Source: CAD feature listing. Evaluate the final solid. Frame: model axes, mm. A direction names the side the tool comes from. Give positions to 0.01 mm unless a question says otherwise; leave off trailing zeros. Loops run counter-clockwise (first coordinate to the right, second up) from the corner with the lowest first, then second, coordinate; pieces in that order, holes last. Notation, with made-up numbers: (64, -6.5) -> (100, -6.5) arc R16 cw to (100, 23.5) -> close; hole circle Ø11 at (-0.5, 19). An arc over 180 degrees is marked (long way). Return JSON: item names as keys, results as strings. Group by question number.
Autodesk Inventor part; units mm, degrees
ref_plane "YZ Plane" through (0, 0, 0) normal (1, 0, 0) x (0, 1, 0)
ref_plane "XZ Plane" through (0, 0, 0) normal (0, 1, 0) x (-1, 0, 0)
ref_plane "XY Plane" through (0, 0, 0) normal (0, 0, 1) x (1, 0, 0)
sketch "Sketch1" plane through (0, 0, 0) normal (0, 0, 1) x (1, 0, 0)
  line L0 (47.0185, 51.5544) -> (-48.0003, 51.5544)
  line L1 (-48.0003, 51.5544) -> (-48.0003, -51.5544)
  line L2 (-48.0003, -51.5544) -> (47.0185, -51.5544)
  line L3 (47.0185, -51.5544) -> (47.0185, 51.5544)
  line L4 (41.2041, -35.74) -> (41.2041, 35.74)
  arc A0 (41.2041, 35.74) -> (31.2041, 45.74) centre (31.2041, 35.74) ccw
  line L5 (31.2041, 45.74) -> (-32.1859, 45.74)
  arc A1 (-32.1859, 45.74) -> (-42.1859, 35.74) centre (-32.1859, 35.74) ccw
  line L6 (-42.1859, 35.74) -> (-42.1859, -35.74)
  arc A2 (-42.1859, -35.74) -> (-32.1859, -45.74) centre (-32.1859, -35.74) ccw
  line L7 (-32.1859, -45.74) -> (31.2041, -45.74)
  arc A3 (31.2041, -45.74) -> (41.2041, -35.74) centre (31.2041, -35.74) ccw
  circle A4 centre (24.0591, 16.9245) radius 1.25
  circle A5 centre (24.0591, -43.0755) radius 1.25
  circle A6 centre (-25.0409, -43.0755) radius 1.25
  circle A7 centre (-25.0409, 16.9245) radius 1.25
  line L8 (25.5091, 38.0745) -> (-26.4909, 38.0745)
  arc A8 (-26.4909, 38.0745) -> (-28.4909, 36.0745) centre (-26.4909, 36.0745) ccw
  line L9 (-28.4909, 36.0745) -> (-28.4909, -44.9255)
  arc A9 (-28.4909, -44.9255) -> (-26.4909, -46.9255) centre (-26.4909, -44.9255) ccw
  line L10 (-26.4909, -46.9255) -> (25.5091, -46.9255)
  arc A10 (25.5091, -46.9255) -> (27.5091, -44.9255) centre (25.5091, -44.9255) ccw
  line L11 (27.5091, -44.9255) -> (27.5091, 36.0745)
  arc A11 (27.5091, 36.0745) -> (25.5091, 38.0745) centre (25.5091, 36.0745) ccw
  point P0 (0, 0)
  dimension "d2" = 5.8144
  dimension "d3" = 5.8144
  dimension "d4" = 5.8144
  dimension "d5" = 5.8144
extrude "Extrusion1" add sketch "Sketch1" along normal blind 3 contours L3 L2 L1 L0 | A3 L7 A10 L11 A11 L8 A8 L9 A9 A2 L6 A1 L5 A0 L4 | A10 L10 A9 L7 | L7 A9 L9 A8 L8 A11 L11 A10 | A4 | A5 | A6 | A7
sketch "Sketch3" plane through (0, 0, 0) normal (0, 0, -1) x (-1, 0, 0)
  line L0 (-41.2041, 35.74) -> (-41.2041, -35.74)
  arc A0 (-41.2041, -35.74) -> (-31.2041, -45.74) centre (-31.2041, -35.74) ccw
  line L1 (-31.2041, -45.74) -> (32.1859, -45.74)
  arc A1 (32.1859, -45.74) -> (42.1859, -35.74) centre (32.1859, -35.74) ccw
  line L2 (42.1859, -35.74) -> (42.1859, 35.74)
  arc A2 (42.1859, 35.74) -> (32.1859, 45.74) centre (32.1859, 35.74) ccw
  line L3 (32.1859, 45.74) -> (-31.2041, 45.74)
  arc A3 (-31.2041, 45.74) -> (-41.2041, 35.74) centre (-31.2041, 35.74) ccw
  line L4 (43.1859, 43.5544) -> (46.1859, 43.5544)
  line L5 (46.1859, 43.5544) -> (46.1859, -43.5544)
  line L6 (46.1859, -43.5544) -> (43.1859, -43.5544)
  line L7 (43.1859, -43.5544) -> (43.1859, 43.5544)
  line L8 (-42.2041, 43.5544) -> (-45.2041, 43.5544)
  line L9 (-45.2041, 43.5544) -> (-45.2041, -43.5544)
  line L10 (-45.2041, -43.5544) -> (-42.2041, -43.5544)
  line L11 (-42.2041, -43.5544) -> (-42.2041, 43.5544)
  line L12 (40.0003, 49.74) -> (-39.0185, 49.74)
  line L13 (-39.0185, 49.74) -> (-39.0185, 46.74)
  line L14 (-39.0185, 46.74) -> (40.0003, 46.74)
  line L15 (40.0003, 46.74) -> (40.0003, 49.74)
  line L16 (40.0003, -46.74) -> (-39.0185, -46.74)
  line L17 (-39.0185, -46.74) -> (-39.0185, -49.74)
  line L18 (-39.0185, -49.74) -> (40.0003, -49.74)
  line L19 (40.0003, -49.74) -> (40.0003, -46.74)
  line L20 (-47.0185, 51.5544) -> (48.0003, 51.5544)
  line L21 (48.0003, 51.5544) -> (48.0003, -51.5544)
  line L22 (48.0003, -51.5544) -> (-47.0185, -51.5544)
  line L23 (-47.0185, -51.5544) -> (-47.0185, 51.5544)
  point P0 (0, 0)
  dimension "d20" = 3
  dimension "d21" = 1
  dimension "d24" = 3
  dimension "d25" = 1
  dimension "d28" = 3
  dimension "d29" = 1
  dimension "d34" = 1
  dimension "d35" = 3
  dimension "d78" = 8
  dimension "d79" = 8
  dimension "d80" = 8
  dimension "d81" = 8
  dimension "d82" = 8
  dimension "d83" = 8
  dimension "d84" = 8
  dimension "d85" = 8
extrude "Extrusion2" add sketch "Sketch3" along normal blind 5 contours L4 L5 L6 L7 | L11 L10 L9 L8 | L15 L14 L13 L12 | L19 L18 L17 L16
sketch "Sketch6" plane through (0, 0, 0) normal (0, 0, -1) x (-1, 0, 0)
  line L0 (48.0003, 51.5544) -> (48.0003, -51.5544)
  line L1 (48.0003, 51.5544) -> (40.0003, 51.5544)
  line L2 (40.0003, 51.5544) -> (40.0003, 43.5544)
  line L3 (40.0003, 43.5544) -> (48.0003, 43.5544)
  line L4 (48.0003, 43.5544) -> (48.0003, 51.5544)
  line L5 (48.0003, -51.5544) -> (40.0003, -51.5544)
  line L6 (40.0003, -51.5544) -> (40.0003, -43.5544)
  line L7 (40.0003, -43.5544) -> (48.0003, -43.5544)
  line L8 (48.0003, -43.5544) -> (48.0003, -51.5544)
  line L9 (48.0003, -51.5544) -> (-47.0185, -51.5544)
  line L10 (-47.0185, -51.5544) -> (-39.0185, -51.5544)
  line L11 (-39.0185, -51.5544) -> (-39.0185, -43.5544)
  line L12 (-39.0185, -43.5544) -> (-47.0185, -43.5544)
  line L13 (-47.0185, -43.5544) -> (-47.0185, -51.5544)
  line L14 (-47.0185, 51.5544) -> (48.0003, 51.5544)
  line L15 (-47.0185, 51.5544) -> (-39.0185, 51.5544)
  line L16 (-39.0185, 51.5544) -> (-39.0185, 43.5544)
  line L17 (-39.0185, 43.5544) -> (-47.0185, 43.5544)
  line L18 (-47.0185, 43.5544) -> (-47.0185, 51.5544)
  point P0 (0, 0)
  dimension "d38" = 8
  dimension "d39" = 8
  dimension "d40" = 8
  dimension "d41" = 8
  dimension "d42" = 8
  dimension "d43" = 8
  dimension "d44" = 8
  dimension "d45" = 8
extrude "Extrusion3" add sketch "Sketch6" along normal blind 6
sketch "Sketch7" plane through (0, 0, 3) normal (0, 0, 1) x (1, 0, 0)
  line L0 (47.0185, -51.5544) -> (47.0185, 51.5544)
  line L1 (47.0185, 51.5544) -> (40.0185, 51.5544)
  line L2 (40.0185, 51.5544) -> (40.0185, 44.5544)
  line L3 (40.0185, 44.5544) -> (47.0185, 44.5544)
  line L4 (47.0185, 44.5544) -> (47.0185, 51.5544)
  line L5 (47.0185, -51.5544) -> (40.0185, -51.5544)
  line L6 (40.0185, -51.5544) -> (40.0185, -44.5544)
  line L7 (40.0185, -44.5544) -> (47.0185, -44.5544)
  line L8 (47.0185, -44.5544) -> (47.0185, -51.5544)
  line L9 (-48.0003, 51.5544) -> (-48.0003, -51.5544)
  line L10 (-48.0003, -51.5544) -> (-41.0003, -51.5544)
  line L11 (-41.0003, -51.5544) -> (-41.0003, -44.5544)
  line L12 (-41.0003, -44.5544) -> (-48.0003, -44.5544)
  line L13 (-48.0003, -44.5544) -> (-48.0003, -51.5544)
  line L14 (-48.0003, 51.5544) -> (-41.0003, 51.5544)
  line L15 (-41.0003, 51.5544) -> (-41.0003, 44.5544)
  line L16 (-41.0003, 44.5544) -> (-48.0003, 44.5544)
  line L17 (-48.0003, 44.5544) -> (-48.0003, 51.5544)
  point P0 (0, 0)
  dimension "d48" = 7
  dimension "d49" = 7
  dimension "d50" = 7
  dimension "d51" = 7
  dimension "d52" = 7
  dimension "d53" = 7
  dimension "d54" = 7
  dimension "d55" = 7
extrude "Extrusion4" cut sketch "Sketch7" against normal blind 6
sketch "Sketch8" plane through (0, 0, -3) normal (0, 0, 1) x (1, 0, 0)
  circle A0 centre (43.5185, 48.0544) radius 1.5
  circle A1 centre (43.5185, -48.0544) radius 1.5
  circle A2 centre (-44.5003, -48.0544) radius 1.5
  circle A3 centre (-44.5003, 48.0544) radius 1.5
  line L0 (47.0185, 51.5544) -> (47.0185, 44.5544)
  line L1 (40.0185, 51.5544) -> (47.0185, 51.5544)
  line L2 (47.0185, -44.5544) -> (47.0185, -51.5544)
  line L3 (47.0185, -51.5544) -> (40.0185, -51.5544)
  line L4 (-48.0003, -51.5544) -> (-48.0003, -44.5544)
  line L5 (-41.0003, -51.5544) -> (-48.0003, -51.5544)
  line L6 (-48.0003, 44.5544) -> (-48.0003, 51.5544)
  line L7 (-48.0003, 51.5544) -> (-41.0003, 51.5544)
  point P0 (0, 0)
  dimension "d58" = 3
  dimension "d59" = 3
  dimension "d60" = 3
  dimension "d61" = 3
  dimension "d62" = 3.5
  dimension "d63" = 3.5
  dimension "d64" = 3.5
  dimension "d65" = 3.5
  dimension "d66" = 3.5
  dimension "d67" = 3.5
  dimension "d68" = 3.5
  dimension "d69" = 3.5
extrude "Extrusion5" cut sketch "Sketch8" against normal up to next
sketch "Sketch9" plane through (0, 0, 3) normal (0, 0, 1) x (1, 0, 0)
  circle A0 centre (24.0497, -29.5956) radius 1.25
  circle A1 centre (-25.0503, -29.5956) radius 1.25
  line L0 (25.4997, 51.5544) -> (-26.5003, 51.5544)
  arc A2 (-26.5003, 51.5544) -> (-28.5003, 49.5544) centre (-26.5003, 49.5544) ccw
  line L1 (-28.5003, 49.5544) -> (-28.5003, -31.4456)
  arc A3 (-28.5003, -31.4456) -> (-26.5003, -33.4456) centre (-26.5003, -31.4456) ccw
  line L2 (-26.5003, -33.4456) -> (25.4997, -33.4456)
  arc A4 (25.4997, -33.4456) -> (27.4997, -31.4456) centre (25.4997, -31.4456) ccw
  line L3 (27.4997, -31.4456) -> (27.4997, 49.5544)
  arc A5 (27.4997, 49.5544) -> (25.4997, 51.5544) centre (25.4997, 49.5544) ccw
  circle A6 centre (24.0497, -29.5956) radius 1.5
  circle A7 centre (-25.0503, -29.5956) radius 1.5
  circle A8 centre (24.0497, 27.9044) radius 1.25
  circle A9 centre (24.0497, -29.5956) radius 1.25
  circle A10 centre (-25.0503, -29.5956) radius 1.25
  circle A11 centre (-25.0503, 27.9044) radius 1.25
  line L4 (25.4997, 51.5544) -> (-26.5003, 51.5544)
  arc A12 (-26.5003, 51.5544) -> (-28.5003, 49.5544) centre (-26.5003, 49.5544) ccw
  line L5 (-28.5003, 49.5544) -> (-28.5003, -31.4456)
  arc A13 (-28.5003, -31.4456) -> (-26.5003, -33.4456) centre (-26.5003, -31.4456) ccw
  line L6 (-26.5003, -33.4456) -> (25.4997, -33.4456)
  arc A14 (25.4997, -33.4456) -> (27.4997, -31.4456) centre (25.4997, -31.4456) ccw
  line L7 (27.4997, -31.4456) -> (27.4997, 49.5544)
  arc A15 (27.4997, 49.5544) -> (25.4997, 51.5544) centre (25.4997, 49.5544) ccw
  circle A16 centre (24.0497, 27.9044) radius 1.5
  circle A17 centre (-25.0503, 27.9044) radius 1.5
  point P0 (0, 0)
  dimension "d73" = 3
  dimension "d74" = 3
  dimension "d86" = 3
  dimension "d87" = 3
extrude "Extrusion6" cut sketch "Sketch9" against normal up to next contours A0 | A1 | A6 | A7 | A8 | A11 | A16 | A17
equation "\"d3\" = d2"
equation "\"d4\" = d2"
equation "\"d5\" = d2"
equation "\"d39\" = d38"
equation "\"d40\" = d38"
equation "\"d41\" = d38"
equation "\"d42\" = d38"
equation "\"d43\" = d38"
equation "\"d44\" = d38"
equation "\"d45\" = d38"
equation "\"d49\" = d48"
equation "\"d50\" = d48"
equation "\"d51\" = d48"
equation "\"d52\" = d48"
equation "\"d53\" = d48"
equation "\"d54\" = d48"
equation "\"d55\" = d48"
equation "\"d62\" = 0.5 * d48"
equation "\"d63\" = d62"
equation "\"d64\" = d62"
equation "\"d65\" = d62"
equation "\"d66\" = d62"
equation "\"d67\" = d62"
equation "\"d68\" = d62"
equation "\"d69\" = d62"
equation "\"d74\" = d73"
equation "\"d86\" = d73"
equation "\"d87\" = d73"
properties part number "akksi-raspi"
1) Contact query for flat-ended pins moving along their axis: P1, Ø1.8, axis at x = 43.52, y = -48.05, coming from the +Z side; P2, Ø1, axis at y = -28, z = -2, coming from the -X side; P3, Ø3.5, axis at x = -17, y = -48.5, coming from the -Z side; P4, Ø2, axis at x = -35, z = -4, coming from the -Y side. Output: stop coordinate, or through.
2) Material intervals for line 1 (X direction, y = 5, z = -1); line 2 (Y direction, x = 18, z = -4.75); line 3 (Y direction, x = 23, z = 2), sorted ascending.
3) Reachability of faces 4 (the face through (43, 50, -3)), 5 (the face through (42.204, -1, -2)), 6 (the face through (0, -49.74, -2)) from +Z, -Z, +X, -X, +Y, -Y: full face, straight path, thin tool, end or side. Return the list, or none.
4) Cut plane B-B on x = 6.5. Return loops of the section in (y, z), then the cut area to 3 significant figures.
5) Cut plane A-A on y = -20.5. Return loops of the section in (x, z).
6) Cut plane C-C on z = 1.5. Return loops of the section in (x, y), then the cut area to 3 significant figures.
7) Mould query, pull axis Y, two halves, no side actions, for faces 1 (the face through (-44, -44.554, 0)), 2 (the face through (-43, -47, -6)), 3 (the face through (45.204, 1, -2)). Classes: released by +Y, released by -Y, zero draft, split by the parting line, or undercut.
Calculated:
{
 "1": {"P1": "through", "P2": "x = -46.19", "P3": "z = -5", "P4": "y = -49.74"},
 "2": {"line 1": "-46.19 to -43.19, 42.2 to 45.2", "line 2": "-49.74 to -46.74, 46.74 to 49.74", "line 3": "-51.55 to -30.67, -28.52 to 26.83, 28.98 to 51.55"},
 "3": {"face 4": "+Z, +X, +Y", "face 5": "-Z", "face 6": "-Z, -Y"},
 "4": {"outline": "(-51.55, 0) -> (-49.74, 0) -> (-49.74, -5) -> (-46.74, -5) -> (-46.74, 0) -> (46.74, 0) -> (46.74, -5) -> (49.74, -5) -> (49.74, 0) -> (51.55, 0) -> (51.55, 3) -> (-51.55, 3) -> close", "area": "339 mm2"},
 "5": {"outline": "(-48, 0) -> (-46.19, 0) -> (-46.19, -5) -> (-43.19, -5) -> (-43.19, 0) -> (42.2, 0) -> (42.2, -5) -> (45.2, -5) -> (45.2, 0) -> (47.02, 0) -> (47.02, 3) -> (-48, 3) -> close"},
 "6": {"outline": "(-48, -44.55) -> (-41, -44.55) -> (-41, -51.55) -> (40.02, -51.55) -> (40.02, -44.55) -> (47.02, -44.55) -> (47.02, 44.55) -> (40.02, 44.55) -> (40.02, 51.55) -> (-41, 51.55) -> (-41, 44.55) -> (-48, 44.55) -> close; hole circle Ø3 at (-25.05, -29.6); hole circle Ø3 at (-25.05, 27.9); hole circle Ø3 at (24.05, -29.6); hole circle Ø3 at (24.05, 27.9)", "area": "9,570 mm2"},
 "7": {"face 1": "released by -Y", "face 2": "zero draft", "face 3": "undercut"}
}
